The listing builds one solid part. Answer for the finished solid, in the listing's coordinates (mm). Face numbers are marked on the shaded views. A direction names the side the tool comes from. Round coordinates to 2 decimals unless told otherwise and drop trailing zeros. Write each loop counter-clockwise with the first axis right and the second up, starting at its lowest first coordinate (ties: lowest second). Pieces come first, ordered by that corner, then holes. Notation, with made-up numbers: (60, 44.25) - (81, 44.25) arc R4 ccw to (81, 48.25) - close; hole circle Ø3 at (64, -6). An arc over 180 degrees is marked (long way). Use a Markdown table: item, result. Add a question column.
1) A cutting plane is placed at B-B (y = 17.78). Give the vertices of the cut face in (x, z) (3 decimals).
2) Each of these flat-tipped pins is pushed along its axis until it touches: P1, Ø3, axis at x = 13, y = -20.5, coming from the -Z side; P2, Ø3, axis at x = 0, y = 16.5, coming from the -Z side; P3, Ø1.5, axis at x = 12.5, z = 2, coming from the -Y side. Where does it stop, or does it pass through?
3) Find the intervals of material crossed by probe 1 along Y at (x, z) = (4, 3.75) (3 decimals); probe 2 along Z at (x, y) = (-11, 19) (3 decimals); probe 3 along Z at (x, y) = (7, -26), in increasing order. Write a range as from..to.
4) A cutting plane is placed at C-C (x = -10). Give the vertices of the cut face in (y, z) (1 decimal).
5) A tool of negligible diameter and unlimited length cuts with its end or side. For the marked faces 1, 2, 3 and 4, from which of +Z, -Z, +X, -X, +Y, -Y can it reach the whole face along a straight path? Write none if from no direction.
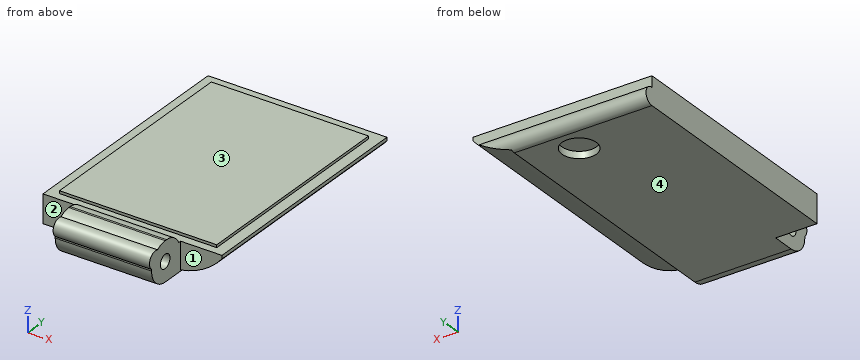
```python
from build123d import *

# Parameters (mm, degrees)
F0_W         = 33.02
F0_H         = 44.45
F1_DEPTH     = 5.715
F2_W         = 17.78
F2_H         = 7.239
F3_DEPTH     = 7.239
F4_R         = 1.27
F5_DEPTH     = 19.05
F6_W         = 33.02
F6_H         = 44.45
F6_W_2       = 29.02
F6_H_2       = 40.45
F7_DEPTH     = 0.5
F9_DEPTH     = 33.02
F10_T1_DEPTH = 35.8775
F10_T3_DEPTH = 34.0243528649
F11_R        = 3.175
F12_DEPTH    = 1.27
F14_DEPTH    = 17.78
F15_W        = 7.62
F15_H        = 5.215
F16_DEPTH    = 0.508
F19_DEPTH    = 76.2


# Not quite as in the source:
# - a fillet or chamfer that OpenCascade refuses, or shapes differently, is made with other operations: its cross-section is extruded or revolved along the edge and cut away or added


with BuildPart() as f1:
    # F0 (on Top) → F1 (new body)
    with BuildSketch(Plane.XY):
        Rectangle(F0_W, F0_H)
    extrude(amount=F1_DEPTH)

    # F2 (on face) → F3 (join)
    with BuildSketch(Plane.XZ.offset(22.225)):
        with Locations((0, 3.6195)):
            Rectangle(F2_W, F2_H)
    extrude(amount=F3_DEPTH)

    # F4 (on face) → F5 (cut)
    with BuildSketch(Plane.YZ.offset(8.89)):
        with Locations((-25.8445, 3.6195)):
            Circle(F4_R)
    extrude(amount=-F5_DEPTH, mode=Mode.SUBTRACT)

    # F6 (on face) → F7 (cut)
    with BuildSketch(Plane.XY.offset(5.715)):
        Rectangle(F6_W, F6_H)
        Rectangle(F6_W_2, F6_H_2, mode=Mode.SUBTRACT)
    extrude(amount=-F7_DEPTH, mode=Mode.SUBTRACT)

    # F8 (on face) → F9 (join, through all)
    with BuildSketch(Plane.YZ.offset(16.51)):
        with BuildLine():
            Line((22.225, 3.175), (22.225, 0))
            ThreePointArc((22.225, 0), (23.8125, 1.5875), (22.225, 3.175))
        make_face()
    extrude(amount=-F9_DEPTH)

    # F10: fillet of radius 3.6195 on 3 edges, made by hand

    # F10_s2 → F10_t1 (cut)
    with BuildSketch(Plane.YZ.offset(-17.93875)):
        with BuildLine():
            ThreePointArc((-29.464, 3.6195), (-28.4038729945, 6.1788729945), (-25.8445, 7.239))
            Line((-25.8445, 7.239), (-25.8445, 7.31139))
            Line((-25.8445, 7.31139), (-29.53639, 7.31139))
            Line((-29.53639, 7.31139), (-29.53639, 3.6195))
            Line((-29.53639, 3.6195), (-29.464, 3.6195))
        make_face()
        with BuildLine():
            ThreePointArc((-25.8445, 0), (-28.4038729945, 1.0601270055), (-29.464, 3.6195))
            Line((-29.464, 3.6195), (-29.53639, 3.6195))
            Line((-29.53639, 3.6195), (-29.53639, -0.07239))
            Line((-29.53639, -0.07239), (-25.8445, -0.07239))
            Line((-25.8445, -0.07239), (-25.8445, 0))
        make_face()
    extrude(amount=F10_T1_DEPTH, mode=Mode.SUBTRACT)

    # F10_s4 → F10_t3 (cut)
    with BuildSketch(Plane.YZ.offset(-17.0121764325)):
        with BuildLine():
            ThreePointArc((-22.225, 5.215), (-23.5599912664, 6.6916077862), (-25.473870573, 7.239))
            Line((-25.473870573, 7.239), (-25.473870573, 7.31139))
            Line((-25.473870573, 7.31139), (-22.225, 7.31139))
            Line((-22.225, 7.31139), (-22.15261, 7.239))
            ThreePointArc((-22.15261, 7.239), (-22.15261, 6.227), (-22.1600225885, 5.24691))
            Line((-22.1600225885, 5.24691), (-22.225, 5.215))
        make_face()
    extrude(amount=F10_T3_DEPTH, mode=Mode.SUBTRACT)

    # F11 (on face) → F12 (cut)
    with BuildSketch(Plane(origin=(0, 0, 0), x_dir=(1, 0, 0), z_dir=(0, 0, -1))):
        with Locations((0, -17.78)):
            Circle(F11_R)
    extrude(amount=-F12_DEPTH, mode=Mode.SUBTRACT)

    # F13 (on face) → F14 (join)
    with BuildSketch(Plane.YZ.offset(8.89)):
        with BuildLine():
            ThreePointArc((-29.4532143561, 3.8987148746), (-28.979078949, 5.42925), (-27.8906643526, 6.6051308701))
            ThreePointArc((-27.8906643526, 6.6051308701), (-29.8039681461, 5.9055), (-29.4532143561, 3.8987148746))
        make_face()
    extrude(amount=-F14_DEPTH)

    # F15 (on face) → F16 (cut)
    with BuildSketch(Plane.XZ.offset(22.225)):
        with Locations((-12.7, 2.6075)):
            Rectangle(F15_W, F15_H)
        with Locations((12.7, 2.6075)):
            Rectangle(F15_W, F15_H)
    extrude(amount=-F16_DEPTH, mode=Mode.SUBTRACT)

    # F18 (on face) → F19 (cut)
    with BuildSketch(Plane.XZ.offset(21.717)):
        with BuildLine():
            ThreePointArc((16.51, 4.5832213708), (13.0932734681, 1.702037729), (8.89, 0.182915771))
            Line((8.89, 0.182915771), (8.89, 0))
            Line((8.89, 0), (16.51, 0))
            Line((16.51, 0), (16.51, 4.5832213708))
        make_face()
    extrude(amount=-F19_DEPTH, mode=Mode.SUBTRACT)


solid = f1.part
```
Entries:
| question | item | result |
|---|---|---|
| 1 | outline | (-16.51, 0) - (-3.175, 0) - (-3.175, 1.27) - (3.175, 1.27) - (3.175, 0) - (8.89, 0) - (8.89, 0.183) arc R12.7 ccw to (16.51, 4.583) - (16.51, 5.215) - (14.51, 5.215) - (14.51, 5.715) - (-14.51, 5.715) - (-14.51, 5.215) - (-16.51, 5.215) - close |
| 2 | P1 | stops at z = 0.92 |
| 2 | P2 | stops at z = 1.27 |
| 2 | P3 | stops at y = -21.72 |
| 3 | probe 1 | y = -29.462..-27.108, -24.581..22.225 |
| 3 | probe 2 | z = 0..5.715 |
| 3 | probe 3 | z = 0..2.36, 4.88..7.24 |
| 4 | outline | (-21.7, 0) - (22.2, 0) arc R1.6 ccw to (22.2, 3.2) - (22.2, 5.2) - (20.2, 5.2) - (20.2, 5.7) - (-20.2, 5.7) - (-20.2, 5.2) - (-21.7, 5.2) - close |
| 5 | face 1 | +Z, -Z, +X, -Y |
| 5 | face 2 | +Z, -Z, -X, -Y |
| 5 | face 3 | +Z, +X, -X, +Y |
| 5 | face 4 | -Z, +X, -X, +Y, -Y |
